Model file for the job. Use its own axes, mm. A direction names the side the tool comes from. Give positions to 0.01 mm unless a question says otherwise; leave off trailing zeros. Loops run counter-clockwise (first coordinate to the right, second up) from the corner with the lowest first, then second, coordinate; pieces in that order, holes last. Notation, with made-up numbers: M -8.75,21.5 L 32.25,21.5 A13 ccw 32.25,30.5 Z; hole C 74,6.25 d9. An arc over 180 degrees is marked long. Use CSV: the item, a comma, the result in double quotes. Start each with the question number.
(1) Two-plate mould, pull along Z, no slides. Class faces 4 (the face through (29.795, 30.242, -50.505)), 5 (the face through (2, 19, -65)), 6 (the face through (2.376, 21, -42)): pulls with the +Z half, pulls with the -Z half, needs draft (parallel to the pull), parting line crosses it, or undercut.
(2) Slice it at C-C on y = 30. List the corners of the cut face in (x, z).
(3) Slice it at B-B on x = 15.5. List the corners of the cut face in (y, z), and give its area (3 significant figures).
(4) Flat gauge pins, fed straight in: P1, Ø6, axis at x = 21.5, z = -46.5, coming from the -Y side; P2, Ø11, axis at x = 15.5, z = -21.23, coming from the +Y side; P3, Ø4, axis at y = 25.5, z = -27, coming from the +X side. Where does each tip first touch, or does it go through?
(5) Slice it at A-A on y = 41.5. List the corners of the cut face in (x, z), and give its area (3 significant figures).
(6) Wall check: line 1 along X through (y, z) = (16, -42.5); line 2 along Y through (x, z) = (11, -27); line 3 along Z through (x, y) = (0.65, 30). Give the ranges that are in metal, low to high. Write a range as from..to.
(7) Slice it at D-D on z = -56. List the corners of the cut face in (x, y), and give its area (3 significant figures).
(8) Tool access for faces 1 (the face through (28.624, 21, -42)), 2 (the face through (18.602, 1, -63)), 3 (the face through (0, 14, -46)): list every direction of +Z, -Z, +X, -X, +Y, -Y with a clear straight run to the whole face (end or side of a thin tool).
```python
from build123d import *

# Parameters (mm, degrees)
SKETCH1_R           = 5.5
BOSS_EXTRUDE1_DEPTH = 31
SKETCH2_W           = 26.247455066
SKETCH2_H           = 52.217390052
CUT_EXTRUDE1_DEPTH  = 88.669835177
SKETCH5_R           = 4.688216148
CUT_EXTRUDE2_DEPTH  = 87.036927024


with BuildPart() as part:
    # Sketch1 → Boss-Extrude1 (new body)
    with BuildSketch(Plane(origin=(0, 0, 0), x_dir=(0, 0, -1), z_dir=(1, 0, 0))):
        Polygon((0, 0), (65, 0), (65, 50), align=None)
        with Locations((56, 30)):
            Circle(SKETCH1_R, mode=Mode.SUBTRACT)
    extrude(amount=BOSS_EXTRUDE1_DEPTH)

    # Sketch2 → Cut-Extrude1 (cut, through all)
    with BuildSketch(Plane(origin=(0, 0, -65), x_dir=(-1, 0, 0), z_dir=(0, 0, -1))):
        with Locations((-15.5, 29.030538608)):
            Rectangle(SKETCH2_W, SKETCH2_H)
    extrude(amount=-CUT_EXTRUDE1_DEPTH, mode=Mode.SUBTRACT)

    # Sketch5 → Cut-Extrude2 (cut, through all)
    with BuildSketch(Plane(origin=(0, 2.921843582, 0), x_dir=(1, 0, 0), z_dir=(0, 1, 0))):
        with Locations(Location((15.5, 21.230034951, 0), (0, 0, 180))):
            Circle(SKETCH5_R)
        with BuildLine():
            Line((18.601825243, 76.649312621), (18.601825243, 60.933398058))
            ThreePointArc((18.601825243, 60.933398058), (15.5, 57.831572816), (12.398174757, 60.933398058))
            Line((12.398174757, 60.933398058), (12.398174757, 76.649312621))
            ThreePointArc((12.398174757, 76.649312621), (15.5, 79.751137864), (18.601825243, 76.649312621))
        make_face()
    extrude(amount=-CUT_EXTRUDE2_DEPTH, mode=Mode.SUBTRACT)


solid = part.part
```
Reply:
1,face 4,"undercut"
1,face 5,"pulls with the -Z half"
1,face 6,"needs draft"
2,outline,"M 0,-65 L 2.38,-65 L 2.38,-61.5 L 0,-61.5 Z; M 0,-50.5 L 2.38,-50.5 L 2.38,-39 L 0,-39 Z; M 28.62,-65 L 31,-65 L 31,-61.5 L 28.62,-61.5 Z; M 28.62,-50.5 L 31,-50.5 L 31,-39 L 28.62,-39 Z"
3,outline,"M 0,-57.83 L 2.92,-57.83 L 2.92,-25.92 L 0,-25.92 Z; M 0,-16.54 L 2.92,-16.54 L 2.92,-3.8 L 0,0 Z"
3,area,"136 mm^2"
4,P1,"stops at y = 0"
4,P2,"stops at y = 2.92"
4,P3,"passes through"
5,outline,"M 0,-65 L 2.38,-65 L 2.38,-53.95 L 0,-53.95 Z; M 28.62,-65 L 31,-65 L 31,-53.95 L 28.62,-53.95 Z"
5,area,"52.5 mm^2"
6,line 1,"x = 0..2.38, 28.62..31"
6,line 2,"y = 0..2.92"
6,line 3,"z = -65..-61.5, -50.5..-39"
7,outline,"M 0,0 L 31,0 L 31,24.5 L 28.62,24.5 L 28.62,2.92 L 2.38,2.92 L 2.38,24.5 L 0,24.5 Z; M 0,35.5 L 2.38,35.5 L 2.38,43.08 L 0,43.08 Z; M 28.62,35.5 L 31,35.5 L 31,43.08 L 28.62,43.08 Z"
7,area,"229 mm^2"
8,face 1,"+Z, -Z, +Y"
8,face 2,"-Z, +Y, -Y"
8,face 3,"+Z, -Z, -X, +Y, -Y"
